Check sheet for the modelled part. Datum: model origin and axes. Units: mm. Face numbers are marked on the shaded views. A direction names the side the tool comes from. Give positions to 0.01 mm unless a question says otherwise; leave off trailing zeros. Loops run counter-clockwise (first coordinate to the right, second up) from the corner with the lowest first, then second, coordinate; pieces in that order, holes last. Notation, with made-up numbers: (-36, 16) - (-15, 16) arc R16 cw to (-15, 20) - close; hole circle Ø7 at (15, 78.25). An arc over 180 degrees is marked (long way). Answer in a Markdown table with one row per item. Add a question column.
(1) Draft check along X on the marked faces 4, 5 and 6. Enter one of: released by +X, released by -X, zero draft, split by the parting line, or undercut.
(2) Go/stop test with flat-tipped pins: P1, Ø9.5, axis at x = 5, y = -41, coming from the +Z side; P2, Ø14.5, axis at x = 31, y = -22, coming from the -Z side; P3, Ø6, axis at y = 49.5, z = 35, coming from the -X side. Record where each tip stops, or that it passes through.
(3) Sectioned sample at B-B on x = 5. Enter the section's corners in (y, z), then the cut area to 3 significant figures.
(4) Sectioned sample at C-C on z = 58. Enter the section's corners in (x, y).
(5) Thickness scan on L1, parallel to Y at x = 55, z = 11; L2, parallel to Z at x = 17, y = -50; L3, parallel to X at y = -35, z = 13.5. Record the ranges inside material, lowest first.
(6) Sectioned sample at D-D on z = 98.5. Enter the section's corners in (x, y), then the cut area to 3 significant figures.
(7) Sectioned sample at A-A on y = 20. Enter the section's corners in (x, z), then the cut area to 3 significant figures.
(8) Set-up check for the marked faces 1, 2 and 3: record each of +Z, -Z, +X, -X, +Y, -Y from which the full face is reachable in a straight line by a thin tool's end or side.
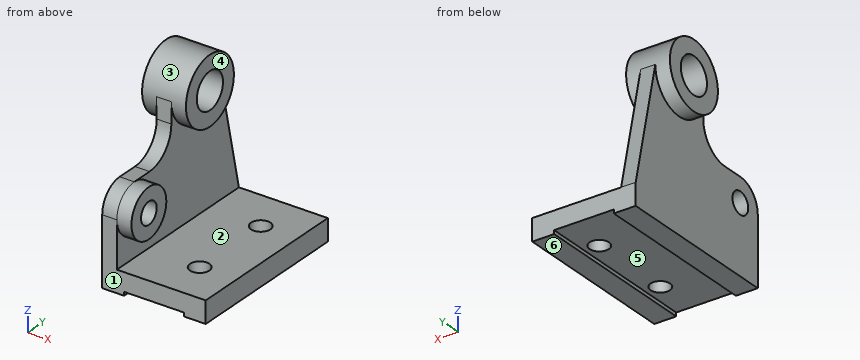
from build123d import *

# Parameters (mm, degrees)
F0_W      = 85
F0_H      = 140
F0_R      = 8
F1_DEPTH  = 18
F2_W      = 49
F2_H      = 3
F3_DEPTH  = 140.001
F4_W      = 12
F4_H      = 140
F5_DEPTH  = 100
F6_R      = 9
F7_DEPTH  = 12
F9_R      = 27.5
F9_R_2    = 15
F10_DEPTH = 18
F11_DEPTH = 25
F12_DEPTH = 25
F13_R     = 25
F14_DEPTH = 25


with BuildPart() as f1:
    # F0 (on Top) → F1 (new body)
    with BuildSketch(Plane.XY):
        with Locations((42.5, 0)):
            Rectangle(F0_W, F0_H)
        with Locations((55, -35)):
            Circle(F0_R, mode=Mode.SUBTRACT)
        with Locations((55, 35)):
            Circle(F0_R, mode=Mode.SUBTRACT)
    extrude(amount=F1_DEPTH)

    # F2 (on face) → F3 (cut, through all)
    with BuildSketch(Plane.XZ.offset(70)):
        with Locations((42.5, 1.5)):
            Rectangle(F2_W, F2_H)
    extrude(amount=-F3_DEPTH, mode=Mode.SUBTRACT)

    # F4 (on face) → F5 (join)
    with BuildSketch(Plane.XY.offset(18)):
        with Locations((6, 0)):
            Rectangle(F4_W, F4_H)
    extrude(amount=F5_DEPTH)

    # F6 (on face) → F7 (join)
    with BuildSketch(Plane.YZ.offset(12)):
        with BuildLine():
            ThreePointArc((-30, 56), (-35.8578643763, 70.1421356237), (-50, 76))
            ThreePointArc((-50, 76), (-64.1421356237, 70.1421356237), (-70, 56))
            ThreePointArc((-70, 56), (-50, 36), (-30, 56))
        make_face()
        with Locations((-50, 56)):
            Circle(F6_R, mode=Mode.SUBTRACT)
    extrude(amount=F7_DEPTH)

    # F9 (on offset) → F10 (join, symmetric)
    with BuildSketch(Plane.YZ.offset(6)):
        with Locations((20, 118)):
            Circle(F9_R)
        with Locations((20, 118)):
            Circle(F9_R_2, mode=Mode.SUBTRACT)
    extrude(amount=F10_DEPTH, both=True)

    # F6 (on face) → F11 (cut)
    with BuildSketch(Plane.YZ.offset(12)):
        with Locations((-50, 56)):
            Circle(F6_R)
        with BuildLine():
            ThreePointArc((5, 118), (20, 103), (35, 118))
            Line((35, 118), (20, 118))
            Line((20, 118), (5, 118))
        make_face()
    extrude(amount=-F11_DEPTH, mode=Mode.SUBTRACT)

    # F6 (on face) → F12 (cut)
    with BuildSketch(Plane.YZ.offset(12)):
        with BuildLine():
            Line((-7.5, 76), (-7.5, 118))
            Line((-7.5, 118), (-70, 118))
            Line((-70, 118), (-70, 56))
            ThreePointArc((-70, 56), (-64.1421356237, 70.1421356237), (-50, 76))
            Line((-50, 76), (-7.5, 76))
        make_face()
        Polygon((70, 118), (47.5, 118), (70, 18), align=None)
    extrude(amount=-F12_DEPTH, mode=Mode.SUBTRACT)

    # F13
    f13_edges = [f1.edges().sort_by_distance(p)[0] for p in [
        (6, -7.5, 76),
    ]]
    fillet(f13_edges, radius=F13_R)

    # F0 (on Top) → F14 (cut)
    with BuildSketch(Plane.XY):
        with Locations((55, -35)):
            Circle(F0_R)
        with Locations((55, 35)):
            Circle(F0_R)
    extrude(amount=-F14_DEPTH, mode=Mode.SUBTRACT)


solid = f1.part
Reply:
| question | item | result |
|---|---|---|
| 1 | face 4 | released by +X |
| 1 | face 5 | undercut |
| 1 | face 6 | zero draft |
| 2 | P1 | z = 76 |
| 2 | P2 | z = 3 |
| 2 | P3 | x = 0 |
| 3 | outline | (-70, 0) - (70, 0) - (70, 18) - (47.5, 118) arc R27.5 ccw to (-7.5, 118) - (-7.5, 101) arc R25 cw to (-32.5, 76) - (-50, 76) arc R20 ccw to (-70, 56) - close; hole circle Ø18 at (-50, 56); hole circle Ø30 at (20, 118) |
| 3 | area | 13,000 mm^2 |
| 4 | outline | (0, -69.9) - (24, -69.9) - (24, -58.77) - (0, -58.77) - close; (0, -41.23) - (24, -41.23) - (24, -30.1) - (12, -30.1) - (12, 61) - (0, 61) - close |
| 5 | L1 | -70 to -43, -27 to 27, 43 to 70 |
| 5 | L2 | 0 to 18, 36 to 47, 65 to 76 |
| 5 | L3 | 0 to 47, 63 to 85 |
| 6 | outline | (-12, 0.61) - (0, 0.61) - (0, -7.63) - (12, -7.63) - (12, 0.61) - (24, 0.61) - (24, 39.39) - (12, 39.39) - (12, 51.89) - (0, 51.89) - (0, 39.39) - (-12, 39.39) - close |
| 6 | area | 1,640 mm^2 |
| 7 | outline | (-12, 90.5) - (0, 90.5) - (0, 0) - (18, 0) - (18, 3) - (67, 3) - (67, 0) - (85, 0) - (85, 18) - (12, 18) - (12, 90.5) - (24, 90.5) - (24, 103) - (-12, 103) - close; (-12, 133) - (24, 133) - (24, 145.5) - (-12, 145.5) - close |
| 7 | area | 3,150 mm^2 |
| 8 | face 1 | +Z, -Z, +X, -X, -Y |
| 8 | face 2 | +X, +Y, -Y |
| 8 | face 3 | none |
